Build history of the part. All positions in model axes, mm. Face numbers are marked on the shaded views. A direction names the side the tool comes from. Round coordinates to 2 decimals unless told otherwise and drop trailing zeros. Order: outer loops, then holes, each group sorted by start corner. A loop starts at its lowest first (then second) coordinate and runs counter-clockwise, first axis right, second up. Notation, with made-up numbers: M -1,30 L 47,30 A22 ccw 47,52 Z; hole C -1.75,65.25 d9. An arc over 180 degrees is marked long. One line per item, written item: value. Start each with the question number.
Item 1: Band-saw the part on B-B, the plane x = 11. Write the cut outline in (y, z).
Item 2: Band-saw the part on D-D, the plane y = 47.5. Write the cut outline in (x, z).
Item 3: Tool access for the marked faces 1 and 2: list every direction of +Z, -Z, +X, -X, +Y, -Y with a clear straight run to the whole face (end or side of a thin tool).
Item 4: Probe L1, parallel to Z at x = 36.98, y = 0.8; L2, parallel to Z at x = 6.5, y = 13; L3, parallel to Y at x = 46, z = 39.5. List the from-to ranges inside material, lowest first.
Item 5: Pin check, flat tips, straight feed: pin 1 (8 mm diameter, centred on x = 36.98, z = 49.25, fed in from +Y); pin 2 (3 mm diameter, centred on x = 82.5, y = 70, fed in from +Z); pin 3 (3 mm diameter, centred on x = 61, y = 58.5, fed in from +Z). Stop position of each tip, or through.
Item 6: Band-saw the part on C-C, the plane z = 91.25. Write the cut outline in (x, y), then the cut area to 3 significant figures.
Item 7: Band-saw the part on A-A, the plane z = 49.25. Write the cut outline in (x, y).
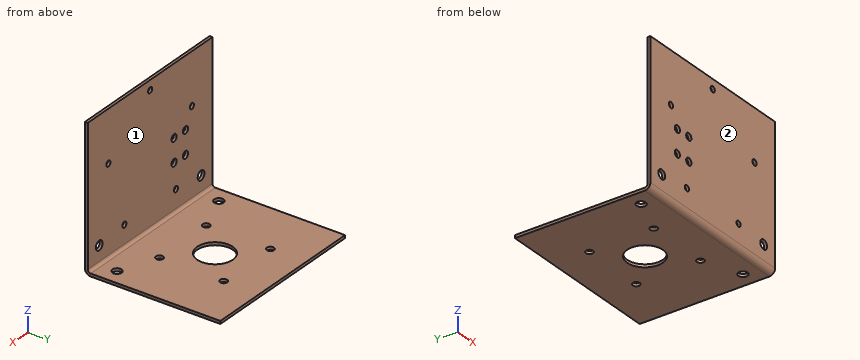
```python
from build123d import *

# Parameters (mm, degrees)
SKETCH2_W                    = 120
SKETCH2_H                    = 95
SKETCH2_R                    = 12.5
SKETCH2_R_2                  = 2.5
SKETCH2_R_3                  = 3.25
BASE_FLANGE1_DEPTH           = 2
EDGE_FLANGE1_STRIP_W         = 12
EDGE_FLANGE1_STRIP_H         = 2
EDGE_FLANGE1_STRIP_CUT_DEPTH = 120
EDGE_FLANGE1_DEPTH           = 120
EDGE_FLANGE1_PROFILE_W       = 120
EDGE_FLANGE1_PROFILE_H       = 96
EDGE_FLANGE1_PROFILE_R       = 3.25
EDGE_FLANGE1_PROFILE_R_2     = 2
EDGE_FLANGE1_PROFILE_R_3     = 2.5
EDGE_FLANGE1_FLAT_DEPTH      = 2


# Sheet-metal steps are written as plain solids
with BuildPart() as part:
    # Sketch2 → Base-Flange1 (new body)
    with BuildSketch(Plane.XY):
        with Locations((60, 47.5)):
            Rectangle(SKETCH2_W, SKETCH2_H)
        with Locations((60, 47.5)):
            Circle(SKETCH2_R, mode=Mode.SUBTRACT)
        with Locations((82.5, 70)):
            Circle(SKETCH2_R_2, mode=Mode.SUBTRACT)
        with Locations((37.5, 70)):
            Circle(SKETCH2_R_2, mode=Mode.SUBTRACT)
        with Locations((37.5, 25)):
            Circle(SKETCH2_R_2, mode=Mode.SUBTRACT)
        with Locations((82.5, 25)):
            Circle(SKETCH2_R_2, mode=Mode.SUBTRACT)
        with Locations((11, 14.5)):
            Circle(SKETCH2_R_3, mode=Mode.SUBTRACT)
        with Locations(Location((109, 14.5, 0), (0, 0, 180))):
            Circle(SKETCH2_R_3, mode=Mode.SUBTRACT)
    extrude(amount=-BASE_FLANGE1_DEPTH)

    # Edge-Flange1 strip (across the edge) → Edge-Flange1 strip cut (cut)
    with BuildSketch(Plane.YZ):
        with Locations((-2, -1)):
            Rectangle(EDGE_FLANGE1_STRIP_W, EDGE_FLANGE1_STRIP_H)
    extrude(amount=EDGE_FLANGE1_STRIP_CUT_DEPTH, mode=Mode.SUBTRACT)

    # Edge-Flange1 bend section (across the edge) → Edge-Flange1 (add)
    with BuildSketch(Plane.YZ):
        with BuildLine():
            Line((0, 2), (2, 2))
            ThreePointArc((2, 2), (2.585786438, 0.585786438), (4, 0))
            Line((4, 0), (4, -2))
            ThreePointArc((4, -2), (1.171572875, -0.828427125), (0, 2))
        make_face()
    extrude(amount=EDGE_FLANGE1_DEPTH)

    # Edge-Flange1 profile (on flange) → Edge-Flange1 flat (add)
    with BuildSketch(Plane.XZ):
        with Locations((60, 50)):
            Rectangle(EDGE_FLANGE1_PROFILE_W, EDGE_FLANGE1_PROFILE_H)
        with Locations((11, 12.5)):
            Circle(EDGE_FLANGE1_PROFILE_R, mode=Mode.SUBTRACT)
        with Locations((35.166073091, 14.819031988)):
            Circle(EDGE_FLANGE1_PROFILE_R_2, mode=Mode.SUBTRACT)
        with Locations((25.98, 33)):
            Circle(EDGE_FLANGE1_PROFILE_R_3, mode=Mode.SUBTRACT)
        with Locations((25.98, 49.25)):
            Circle(EDGE_FLANGE1_PROFILE_R_3, mode=Mode.SUBTRACT)
        with Locations((36.98, 33)):
            Circle(EDGE_FLANGE1_PROFILE_R_3, mode=Mode.SUBTRACT)
        with Locations((36.98, 49.25)):
            Circle(EDGE_FLANGE1_PROFILE_R_3, mode=Mode.SUBTRACT)
        with Locations((84.833926909, 14.819031988)):
            Circle(EDGE_FLANGE1_PROFILE_R_2, mode=Mode.SUBTRACT)
        with Locations((109, 12.5)):
            Circle(EDGE_FLANGE1_PROFILE_R, mode=Mode.SUBTRACT)
        with Locations((19.817862187, 62.055968012)):
            Circle(EDGE_FLANGE1_PROFILE_R_2, mode=Mode.SUBTRACT)
        with Locations((100.182137813, 62.055968012)):
            Circle(EDGE_FLANGE1_PROFILE_R_2, mode=Mode.SUBTRACT)
        with Locations((60, 91.25)):
            Circle(EDGE_FLANGE1_PROFILE_R_2, mode=Mode.SUBTRACT)
    extrude(amount=-EDGE_FLANGE1_FLAT_DEPTH)


solid = part.part
```
Output:
1. outline: M 0,2 A4 ccw 4,-2 L 11.25,-2 L 11.25,0 L 4,0 A2 cw 2,2 L 2,9.25 L 0,9.25 Z; M 0,15.75 L 2,15.75 L 2,98 L 0,98 Z; M 17.75,-2 L 95,-2 L 95,0 L 17.75,0 Z
2. outline: M 0,-2 L 47.5,-2 L 47.5,0 L 0,0 Z; M 72.5,-2 L 120,-2 L 120,0 L 72.5,0 Z
3. face 1: +Z, +X, -X, +Y
3. face 2: +Z, -Z, +X, -X, -Y
4. L1: z = -0.4 to 13.98, 15.66 to 30.5, 35.5 to 46.75, 51.75 to 98
4. L2: z = -2 to 0
4. L3: y = 0 to 2
5. pin 1: stops at y = 2
5. pin 2: passes through
5. pin 3: stops at z = 0
6. outline: M 0,0 L 58,0 L 58,2 L 0,2 Z; M 62,0 L 120,0 L 120,2 L 62,2 Z
6. area: 232 mm²
7. outline: M 0,0 L 23.48,0 L 23.48,2 L 0,2 Z; M 28.48,0 L 34.48,0 L 34.48,2 L 28.48,2 Z; M 39.48,0 L 120,0 L 120,2 L 39.48,2 Z
